Here's how the part is built. I have some questions about the finished solid (model axes, mm). Face numbers are marked on the shaded views. Coordinates: 2 decimals unless noted, no trailing zeros. Order: outer loops, then holes, each group sorted by start corner. A loop starts at its lowest first (then second) coordinate and runs counter-clockwise, first axis right, second up. Notation, with made-up numbers: (62, 61.25) - (118, 61.25) arc R15 ccw to (118, 90.25) - close; hole circle Ø4 at (77, -27.5). An arc over 180 degrees is marked (long way). Use one line per item in the form item = value. Start each with the question number.
from build123d import *

# Parameters (mm, degrees)
SKETCH_W     = 34
SKETCH_H     = 22
SKETCH_R     = 4
PAD_DEPTH    = 30
CHAMFER_SIZE = 5
SKETCH001_R  = 2
POCKET_DEPTH = 22


with BuildPart() as part:
    # Sketch → Pad (new body)
    with BuildSketch(Plane.XZ):
        with Locations((17, 11)):
            Rectangle(SKETCH_W, SKETCH_H)
        with Locations((17, 11)):
            Circle(SKETCH_R, mode=Mode.SUBTRACT)
    extrude(amount=PAD_DEPTH)

    # Chamfer
    chamfer_edges = [part.edges().sort_by_distance(p)[0] for p in [
        (0, -15, 0),
        (34, -15, 0),
    ]]
    chamfer(chamfer_edges, length=CHAMFER_SIZE)

    # Sketch001 (on Face8 of Chamfer) → Pocket (cut)
    with BuildSketch(Plane(origin=(0, 0, 22), x_dir=(-1, 0, 0), z_dir=(0, 0, 1))):
        with Locations((-29, 24)):
            Circle(SKETCH001_R)
        with Locations((-5, 24)):
            Circle(SKETCH001_R)
        with Locations((-29, 6)):
            Circle(SKETCH001_R)
        with Locations((-5, 6)):
            Circle(SKETCH001_R)
    extrude(amount=-POCKET_DEPTH, mode=Mode.SUBTRACT)


solid = part.part
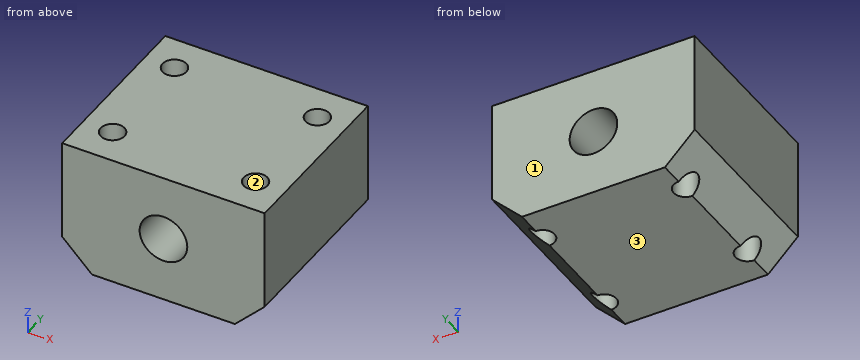
1) Suppose I cut it at D-D, the plane z = 9.25. List the corners of the cut face in (x, y) for me.
2) I need wall thicknesses on probe 1 along X at (y, z) = (-6, 16); probe 2 along Y at (x, z) = (5, 13); probe 3 along X at (y, z) = (-24, 10). Which ranges of each line are inside material? Lowest first, please. Write a range as [from, to].
3) If we mould it in two halves opening along Y, with no side actions, what happens to the marked faces 1, 2 and 3? For each: pulls with the +Y half, pulls with the -Y half, needs draft (parallel to the pull), parting line crosses it, or undercut.
4) For pin 1 (3.5 mm diameter, centred on x = 29, y = -6, fed in from +Z), with a flat end and sliding along its axis, tell me the tip position at first contact or that it passes through.
5) Suppose I cut it at A-A, the plane y = -5. List the corners of the cut face in (x, z) for me, then the cut area to 3 significant figures.
6) Suppose I cut it at B-B, the plane z = 2.5. List the corners of the cut face in (x, y) for me.
7) Suppose I cut it at C-C, the plane x = 17. List the corners of the cut face in (y, z) for me, then the cut area to 3 significant figures.
From the geometry:
q1.outline = (0, -30) - (13.4, -30) - (13.4, 0) - (0, 0) - close; (20.6, -30) - (34, -30) - (34, 0) - (20.6, 0) - close; hole circle Ø4 at (5, -24); hole circle Ø4 at (5, -6); hole circle Ø4 at (29, -24); hole circle Ø4 at (29, -6)
q2.probe_1 = [0, 3], [7, 27], [31, 34]
q2.probe_2 = [-30, -26], [-22, -8], [-4, 0]
q2.probe_3 = [0, 3], [7, 13.13], [20.87, 27], [31, 34]
q3.face_1 = pulls with the +Y half
q3.face_2 = undercut
q3.face_3 = needs draft
q4.pin_1 = through
q5.outline = (0, 5) - (3.27, 1.73) - (3.27, 22) - (0, 22) - close; (6.73, 0) - (27.27, 0) - (27.27, 22) - (6.73, 22) - close; (30.73, 1.73) - (34, 5) - (34, 22) - (30.73, 22) - close; hole circle Ø8 at (17, 11)
q5.area = 523 mm2
q6.outline = (2.5, -30) - (31.5, -30) - (31.5, 0) - (2.5, 0) - close; hole circle Ø4 at (5, -24); hole circle Ø4 at (5, -6); hole circle Ø4 at (29, -24); hole circle Ø4 at (29, -6)
q7.outline = (-30, 0) - (0, 0) - (0, 7) - (-30, 7) - close; (-30, 15) - (0, 15) - (0, 22) - (-30, 22) - close
q7.area = 420 mm2
